Read the model definition and answer for the solid it produces. Units are mm, in the model's axes. A direction names the side the tool comes from. Round coordinates to 2 decimals unless told otherwise and drop trailing zeros. Write each loop counter-clockwise with the first axis right and the second up, starting at its lowest first coordinate (ties: lowest second). Pieces come first, ordered by that corner, then holes. Notation, with made-up numbers: (67.25, 71.25) - (97.25, 71.25) arc R33 ccw to (97.25, 102.25) - close; hole circle Ø9 at (2, -6.75). An arc over 180 degrees is marked (long way). One line per item, written item: value. Start each with the question number.
(1) Flat-ended cylindrical pins translate along their axes: pin 1 Ø3 at (x, z) = (-1, -9.5) entering from -Y; pin 2 Ø0.9 at (y, z) = (-1, 10.5) entering from -X; pin 3 Ø1 at (y, z) = (-2.5, 35.5) entering from -X. Find the tip coordinate at first contact, or state that the pin passes through.
(2) A cutting plane is placed at A-A, the plane y = -0.7. Determine the outline of the cut face in (x, z), plus the area to 4 significant figures.
(3) A cutting plane is placed at C-C, the plane z = -20.5. Determine the outline of the cut face in (x, y), plus the area to 3 significant figures.
(4) A cutting plane is placed at B-B, the plane x = 4. Determine the outline of the cut face in (y, z), plus the area to 3 significant figures.
(5) The mould has two halves that part along Z. Classify faces 1 (the face through (1, -1, -33.5)), 2 (the face through (1, -4, 36)), 3 (the face through (-4.9, 0.99, 36.43)), 4 (the face through (1, -2, 35)): +Z half, -Z half, draft (parallel to the pull), parting line (faces both ways), or undercut.
(6) For faces 5 (the face through (-4, -1, 0)), 6 (the face through (-3.5, -2, 36)), 7 (the face through (1, -3, 0)), 8 (the face through (1, -1, 33.5)), 9 (the face through (-4.93, 1.01, -34.4)), determine the directions among +Z, -Z, +X, -X, +Y, -Y from which every point of the face is accessible in a straight line to the end or side of a thin tool.
(7) Find the intervals of material crossed by L1, parallel to Z at x = 2.75, y = -1.2; L2, parallel to Z at x = 5, y = -3.1; L3, parallel to X at y = -1.45, z = 23, in increasing order.
from build123d import *

# Parameters (mm, degrees)
EXTRUDE_1_DEPTH     = 2
SKETCH_2_W          = 9
SKETCH_2_H          = 2
EXTRUDE_2_DEPTH     = 4
SKETCH_3_W          = 9.5
SKETCH_3_H          = 67
EXTRUDE_3_DEPTH     = 3
SKETCH_4_W          = 16.00447387
SKETCH_4_H          = 2
CUT_EXTRUDE_1_DEPTH = 10
FILLET_1_R          = 2


with BuildPart() as part:
    # 草图1 → 凸台-拉伸1 (new body)
    with BuildSketch(Plane(origin=(0, 0, 0), x_dir=(1, 0, 0), z_dir=(0, 1, 0))):
        with BuildLine():
            Line((-3.5, 37), (5.5, 37))
            Line((5.5, 37), (5.5, -37))
            Line((5.5, -37), (-3.5, -37))
            ThreePointArc((-3.5, -37), (-4.914213562, -36.414213562), (-5.5, -35))
            Line((-5.5, -35), (-5.5, 35))
            ThreePointArc((-5.5, 35), (-4.914213562, 36.414213562), (-3.5, 37))
        make_face()
    extrude(amount=EXTRUDE_1_DEPTH)

    # 草图2 → 凸台-拉伸2 (add)
    with BuildSketch(Plane.XZ):
        with Locations((1, 36)):
            Rectangle(SKETCH_2_W, SKETCH_2_H)
        with Locations((1, -36)):
            Rectangle(SKETCH_2_W, SKETCH_2_H)
    extrude(amount=EXTRUDE_2_DEPTH)

    # 草图3 → 凸台-拉伸3 (add)
    with BuildSketch(Plane.XZ):
        with Locations((0.75, 0)):
            Rectangle(SKETCH_3_W, SKETCH_3_H)
    extrude(amount=EXTRUDE_3_DEPTH)

    # 草图4 → 切除-拉伸1 (cut)
    with BuildSketch(Plane.XZ.offset(4)):
        with Locations((-2.502236935, -36)):
            Rectangle(SKETCH_4_W, SKETCH_4_H)
    extrude(amount=-CUT_EXTRUDE_1_DEPTH, mode=Mode.SUBTRACT)

    # 圆角1
    fillet_1_edges = [part.edges().sort_by_distance(p)[0] for p in [
        (-5.5, 1, -35),
    ]]
    fillet(fillet_1_edges, radius=FILLET_1_R)


solid = part.part
Here are the results:
1. pin 1: y = -3
1. pin 2: x = -4
1. pin 3: x = -3.5
2. outline: (-4, -33.5) - (5.5, -33.5) - (5.5, 33.5) - (-4, 33.5) - close; (-3.5, 35) - (5.5, 35) - (5.5, 37) - (-3.5, 37) - close
2. area: 654.5 mm²
3. outline: (-5.5, 0) - (-4, 0) - (-4, -3) - (5.5, -3) - (5.5, 2) - (-5.5, 2) - close
3. area: 50.5 mm²
4. outline: (-4, 35) - (0, 35) - (0, 33.5) - (-3, 33.5) - (-3, -33.5) - (0, -33.5) - (0, -35) - (2, -35) - (2, 37) - (-4, 37) - close
4. area: 353 mm²
5. face 1: -Z half
5. face 2: draft
5. face 3: +Z half
5. face 4: undercut
6. face 5: +Z, -Z, -X, -Y
6. face 6: +Z, -X, -Y
6. face 7: -Z, +X, -X, -Y
6. face 8: +X, -X, -Y
6. face 9: -Z, -X, +Y, -Y
7. L1: -33.5 to 33.5, 35 to 37
7. L2: 35 to 37
7. L3: -4 to 5.5
